Read the model definition and answer for the solid it produces. Units are mm, in the model's axes. Give positions to 0.01 mm unless a question says otherwise; leave off trailing zeros. Order: outer loops, then holes, each group sorted by start corner. A loop starts at its lowest first (then second) coordinate and runs counter-clockwise, first axis right, second up. Notation, with made-up numbers: (21.5, 0.25) -> (52.5, 0.25) arc R7 ccw to (52.5, 4.25) -> close; hole circle Ø5 at (-38, -31.75). An arc over 180 degrees is marked (long way). One line per item, written item: value. Start each with the question number.
Autodesk Fusion 360 part; units mm, degrees
sketch "Outer" plane through (0, 0, 0) normal (0, 1, 0) x (1, 0, 0)
  circle A0 centre (0, 0) radius 12.5
  dimension "d1" = 25
extrude "Extrude1" add sketch "Outer" along normal blind 20
sketch "Inner" plane through (0, 20, 0) normal (0, 1, 0) x (-1, 0, 0)
  circle A0 centre (0, 0) radius 12.5
  circle A1 centre (0, 0) radius 10.5
  dimension "d4" = 21
extrude "Extrude2" cut sketch "Inner" against normal blind 18 contours A1
sketch "Shaft" plane through (0, 2, 0) normal (0, 1, 0) x (-1, 0, 0)
  circle A0 centre (0, 0) radius 10.5
  line L0 (-1.7, 2.7111) -> (-1.7, -2.7111)
  arc A1 (-1.7, -2.7111) -> (-1.7, 2.7111) centre (0, 0) ccw
  arc A2 (-3.7, -3.6538) -> (-3.7, 3.6538) centre (0, 0) ccw
  line L1 (-3.7, 3.6538) -> (-3.7, -3.6538)
  dimension "d7" = 6.4
  dimension "d8" = 1.7
  dimension "d9" = 2
extrude "Extrude3" add sketch "Shaft" along normal blind 12.5 contours A2 L1
sketch "Sketch4" plane through (0, 2, 0) normal (0, 1, 0) x (-1, 0, 0)
  line L0 (-1.7, 2.7111) -> (-1.7, -2.7111)
  arc A0 (-1.7, -2.7111) -> (-1.7, 2.7111) centre (0, 0) ccw
extrude "Extrude4" add sketch "Sketch4" along normal blind 5
equation "d4 = 25 mm - 2 mm - 2 mm"
equation "d5 = -( 20 mm - 2 mm )"
equation "d7 = 6 mm + 0.2 mm + 0.2 mm"
equation "d8 = ( 4.5 mm - 3 mm ) + 0.2 mm"
equation "d10 = 20 mm - 2 mm - 5.5 mm"
equation "d12 = 20 mm - 2 mm - 5.5 mm - 7.5 mm"
Item 1: Find section C-C on x = 0. Write down the section's boundary in (y, z), then the cut area to 3 significant figures.
Item 2: Find section A-A on y = 11.5. Write down the section's boundary in (x, z), then the cut area to 3 significant figures.
Item 3: Find section B-B on y = 4.5. Write down the section's boundary in (x, z).
Item 4: Find the intervals of material crossed by line 1 (Z direction, x = 0, y = 11.75); line 2 (X direction, y = 5.25, z = 3.5); line 3 (Y direction, x = -3.5, z = 7.5), in increasing order. Write a range as from..to.
Item 5: Flat-ended cylindrical pins translate along their axes: pin 1 (2 mm diameter, centred on x = -1, z = 2, fed in from +Y); pin 2 (1.5 mm diameter, centred on x = -10, y = 13.5, fed in from -Z); pin 3 (3 mm diameter, centred on x = -7.5, y = 5.5, fed in from +Z). Find the tip coordinate at first contact, or state that the pin passes through.
Item 6: For a pull along Z with two mould halves and no side action, classify faces 1 (the cylindrical face through (11.923, 9.86, 3.755)), 2 (the flat face through (2, 14.5, 0)), 3 (the flat face through (0, 0, 0)) as +Z half, -Z half, draft (parallel to the pull), parting line (faces both ways), or undercut.
Item 7: Find section D-D on z = 0. Write down the section's boundary in (x, y).
Checks:
1. outline: (0, -12.5) -> (20, -12.5) -> (20, -10.5) -> (2, -10.5) -> (2, -5.2) -> (14.5, -5.2) -> (14.5, -3.2) -> (7, -3.2) -> (7, 3.2) -> (14.5, 3.2) -> (14.5, 5.2) -> (2, 5.2) -> (2, 10.5) -> (20, 10.5) -> (20, 12.5) -> (0, 12.5) -> close
1. area: 204 mm2
2. outline: circle Ø25 at (0, 0); (3.7, -3.65) -> (3.7, 3.65) arc R5.2 ccw (long way) to start; hole circle Ø21 at (0, 0); hole (1.7, -2.71) -> (1.7, 2.71) arc R3.2 ccw (long way) to start
2. area: 195 mm2
3. outline: circle Ø25 at (0, 0); (3.7, -3.65) -> (3.7, 3.65) arc R5.2 ccw (long way) to start; hole circle Ø21 at (0, 0)
4. line 1: -12.5..-10.5, -5.2..-3.2, 3.2..5.2, 10.5..12.5
4. line 2: -12..-9.9, -3.85..3.7, 9.9..12
4. line 3: 0..2
5. pin 1: y = 14.5
5. pin 2: z = -8.41
5. pin 3: z = 10.97
6. face 1: parting line
6. face 2: undercut
6. face 3: draft
7. outline: (-12.5, 0) -> (12.5, 0) -> (12.5, 20) -> (10.5, 20) -> (10.5, 2) -> (3.7, 2) -> (3.7, 14.5) -> (1.7, 14.5) -> (1.7, 7) -> (-3.2, 7) -> (-3.2, 14.5) -> (-5.2, 14.5) -> (-5.2, 2) -> (-10.5, 2) -> (-10.5, 20) -> (-12.5, 20) -> close
